Part model, mm, in its own coordinate system. Face numbers are marked on the shaded views. Give positions to 0.01 mm unless a question says otherwise; leave off trailing zeros. Order: outer loops, then holes, each group sorted by start corner. A loop starts at its lowest first (then second) coordinate and runs counter-clockwise, first axis right, second up. Notation, with made-up numbers: (9.25, 84) -> (35.25, 84) arc R23 cw to (35.25, 113) -> close; hole circle Ø7 at (27.5, 15.25). An arc over 180 degrees is marked (long way). Write item = value, one per line. Start each with the question number.
(1) Saw through at D-D, the plane y = 1.55. State how many separate pieces and enclosed holes the cut face has, then the cut area to 3 significant figures.
(2) Two-plate mould, pull along Y, no slides. Class the marked faces 1 and 2: pulls with the +Y half, pulls with the -Y half, needs draft (parallel to the pull), parting line crosses it, or undercut.
(3) Saw through at C-C, the plane x = 5. List the corners of the cut face in (y, z), then the cut area to 3 significant figures.
(4) Saw through at B-B, the plane z = 0. List the corners of the cut face in (x, y), then the cut area to 3 significant figures.
(5) Probe line 1 along Z through (x, y) = (160, 1); line 2 along Z through (x, y) = (172.5, 1.1); line 3 along X through (y, z) = (1.6, 4.5). List the from-to ranges inside material, lowest first. Write a range as from..to.
(6) Flat gauge pins, fed straight in: pin 1 (1 mm diameter, centred on y = 1.5, z = 10.5, fed in from -X); pin 2 (0.5 mm diameter, centred on y = 1.5, z = -3.5, fed in from +X); pin 3 (12.5 mm diameter, centred on x = 231.5, z = 2, fed in from +Y). Where does each tip first touch, or does it go through?
(7) Saw through at A-A, the plane x = 220. List the corners of the cut face in (y, z).
from build123d import *

# Parameters (mm, degrees)
BOSS_EXTRUDE1_DEPTH = 1.9
BOSS_EXTRUDE3_DEPTH = 0.95
SKETCH2_W           = 2
SKETCH2_H           = 5
BOSS_EXTRUDE2_DEPTH = 0.95


with BuildPart() as part:
    # Sketch1 → Boss-Extrude1 (new body)
    with BuildSketch(Plane(origin=(0, 0, 0), x_dir=(1, 0, 0), z_dir=(0, 1, 0))):
        with BuildLine():
            Line((0, -7.5), (0, -12.5))
            Line((0, -12.5), (210, -12.5))
            Line((210, -12.5), (210, 12.5))
            Line((210, 12.5), (0, 12.5))
            Line((0, 12.5), (0, 7.5))
            ThreePointArc((0, 7.5), (1.26826484, 7.391989197), (2.5, 7.071067812))
            ThreePointArc((2.5, 7.071067812), (12.5, 0), (2.5, -7.071067812))
            ThreePointArc((2.5, -7.071067812), (1.26826484, -7.391989197), (0, -7.5))
        make_face()
        with BuildLine():
            ThreePointArc((37.5, 7.071067812), (40, 7.5), (42.5, 7.071067812))
            ThreePointArc((42.5, 7.071067812), (45, 7.5), (47.5, 7.071067812))
            ThreePointArc((47.5, 7.071067812), (50, 7.5), (52.5, 7.071067812))
            ThreePointArc((52.5, 7.071067812), (55, 7.5), (57.5, 7.071067812))
            ThreePointArc((57.5, 7.071067812), (60, 7.5), (62.5, 7.071067812))
            ThreePointArc((62.5, 7.071067812), (65, 7.5), (67.5, 7.071067812))
            ThreePointArc((67.5, 7.071067812), (70, 7.5), (72.5, 7.071067812))
            ThreePointArc((72.5, 7.071067812), (75, 7.5), (77.5, 7.071067812))
            ThreePointArc((77.5, 7.071067812), (87.5, 0), (77.5, -7.071067812))
            ThreePointArc((77.5, -7.071067812), (75, -7.5), (72.5, -7.071067812))
            ThreePointArc((72.5, -7.071067812), (70, -7.5), (67.5, -7.071067812))
            ThreePointArc((67.5, -7.071067812), (65, -7.5), (62.5, -7.071067812))
            ThreePointArc((62.5, -7.071067812), (60, -7.5), (57.5, -7.071067812))
            ThreePointArc((57.5, -7.071067812), (55, -7.5), (52.5, -7.071067812))
            ThreePointArc((52.5, -7.071067812), (50, -7.5), (47.5, -7.071067812))
            ThreePointArc((47.5, -7.071067812), (45, -7.5), (42.5, -7.071067812))
            ThreePointArc((42.5, -7.071067812), (40, -7.5), (37.5, -7.071067812))
            ThreePointArc((37.5, -7.071067812), (27.5, 0), (37.5, 7.071067812))
        make_face(mode=Mode.SUBTRACT)
        with BuildLine():
            ThreePointArc((102.5, 7.071067812), (105, 7.5), (107.5, 7.071067812))
            ThreePointArc((107.5, 7.071067812), (110, 7.5), (112.5, 7.071067812))
            ThreePointArc((112.5, 7.071067812), (115, 7.5), (117.5, 7.071067812))
            ThreePointArc((117.5, 7.071067812), (120, 7.5), (122.5, 7.071067812))
            ThreePointArc((122.5, 7.071067812), (125, 7.5), (127.5, 7.071067812))
            ThreePointArc((127.5, 7.071067812), (130, 7.5), (132.5, 7.071067812))
            ThreePointArc((132.5, 7.071067812), (135, 7.5), (137.5, 7.071067812))
            ThreePointArc((137.5, 7.071067812), (147.5, 0), (137.5, -7.071067812))
            ThreePointArc((137.5, -7.071067812), (135, -7.5), (132.5, -7.071067812))
            ThreePointArc((132.5, -7.071067812), (130, -7.5), (127.5, -7.071067812))
            ThreePointArc((127.5, -7.071067812), (125, -7.5), (122.5, -7.071067812))
            ThreePointArc((122.5, -7.071067812), (120, -7.5), (117.5, -7.071067812))
            ThreePointArc((117.5, -7.071067812), (115, -7.5), (112.5, -7.071067812))
            ThreePointArc((112.5, -7.071067812), (110, -7.5), (107.5, -7.071067812))
            ThreePointArc((107.5, -7.071067812), (105, -7.5), (102.5, -7.071067812))
            ThreePointArc((102.5, -7.071067812), (92.5, 0), (102.5, 7.071067812))
        make_face(mode=Mode.SUBTRACT)
        with BuildLine():
            ThreePointArc((162.5, 7.071067812), (165, 7.5), (167.5, 7.071067812))
            ThreePointArc((167.5, 7.071067812), (170, 7.5), (172.5, 7.071067812))
            ThreePointArc((172.5, 7.071067812), (175, 7.5), (177.5, 7.071067812))
            ThreePointArc((177.5, 7.071067812), (180, 7.5), (182.5, 7.071067812))
            ThreePointArc((182.5, 7.071067812), (185, 7.5), (187.5, 7.071067812))
            ThreePointArc((187.5, 7.071067812), (190, 7.5), (192.5, 7.071067812))
            ThreePointArc((192.5, 7.071067812), (195, 7.5), (197.5, 7.071067812))
            ThreePointArc((197.5, 7.071067812), (207.5, 0), (197.5, -7.071067812))
            ThreePointArc((197.5, -7.071067812), (195, -7.5), (192.5, -7.071067812))
            ThreePointArc((192.5, -7.071067812), (190, -7.5), (187.5, -7.071067812))
            ThreePointArc((187.5, -7.071067812), (185, -7.5), (182.5, -7.071067812))
            ThreePointArc((182.5, -7.071067812), (180, -7.5), (177.5, -7.071067812))
            ThreePointArc((177.5, -7.071067812), (175, -7.5), (172.5, -7.071067812))
            ThreePointArc((172.5, -7.071067812), (170, -7.5), (167.5, -7.071067812))
            ThreePointArc((167.5, -7.071067812), (165, -7.5), (162.5, -7.071067812))
            ThreePointArc((162.5, -7.071067812), (152.5, 0), (162.5, 7.071067812))
        make_face(mode=Mode.SUBTRACT)
    extrude(amount=BOSS_EXTRUDE1_DEPTH)

    # Sketch1<3> → Boss-Extrude3 (add)
    with BuildSketch(Plane(origin=(0, 0, 0), x_dir=(1, 0, 0), z_dir=(0, 1, 0))):
        with BuildLine():
            Line((210, -12.5), (245, -12.5))
            ThreePointArc((245, -12.5), (257.5, 0), (245, 12.5))
            Line((245, 12.5), (210, 12.5))
            Line((210, 12.5), (210, -12.5))
        make_face()
        with BuildLine():
            ThreePointArc((222.5, -7.071067812), (212.5, 0), (222.5, 7.071067812))
            ThreePointArc((222.5, 7.071067812), (225, 7.5), (227.5, 7.071067812))
            ThreePointArc((227.5, 7.071067812), (230, 7.5), (232.5, 7.071067812))
            ThreePointArc((232.5, 7.071067812), (235, 7.5), (237.5, 7.071067812))
            ThreePointArc((237.5, 7.071067812), (240, 7.5), (242.5, 7.071067812))
            ThreePointArc((242.5, 7.071067812), (252.5, 0), (242.5, -7.071067812))
            ThreePointArc((242.5, -7.071067812), (240, -7.5), (237.5, -7.071067812))
            ThreePointArc((237.5, -7.071067812), (235, -7.5), (232.5, -7.071067812))
            ThreePointArc((232.5, -7.071067812), (230, -7.5), (227.5, -7.071067812))
            ThreePointArc((227.5, -7.071067812), (225, -7.5), (222.5, -7.071067812))
        make_face(mode=Mode.SUBTRACT)
    extrude(amount=BOSS_EXTRUDE3_DEPTH)

    # Sketch2 → Boss-Extrude2 (add)
    with BuildSketch(Plane(origin=(0, 0, 0), x_dir=(1, 0, 0), z_dir=(0, 1, 0))):
        with Locations((-1, 10)):
            Rectangle(SKETCH2_W, SKETCH2_H)
        with Locations((-1, -10)):
            Rectangle(SKETCH2_W, SKETCH2_H)
    extrude(amount=BOSS_EXTRUDE2_DEPTH)


solid = part.part
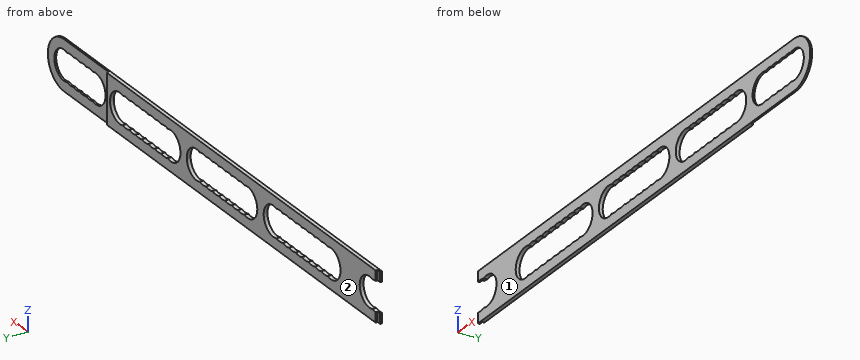
Results list:
q1.separate_pieces = 1
q1.enclosed_holes = 3
q1.area = 2,720 mm^2
q2.face_1 = pulls with the -Y half
q2.face_2 = pulls with the +Y half
q3.outline = (0, -12.5) -> (1.9, -12.5) -> (1.9, -7.5) -> (0, -7.5) -> close; (0, 7.5) -> (1.9, 7.5) -> (1.9, 12.5) -> (0, 12.5) -> close
q3.area = 19.0 mm^2
q4.outline = (12.5, 0) -> (27.5, 0) -> (27.5, 1.9) -> (12.5, 1.9) -> close; (87.5, 0) -> (92.5, 0) -> (92.5, 1.9) -> (87.5, 1.9) -> close; (147.5, 0) -> (152.5, 0) -> (152.5, 1.9) -> (147.5, 1.9) -> close; (207.5, 0) -> (212.5, 0) -> (212.5, 0.95) -> (210, 0.95) -> (210, 1.9) -> (207.5, 1.9) -> close; (252.5, 0) -> (257.5, 0) -> (257.5, 0.95) -> (252.5, 0.95) -> close
q4.area = 59.4 mm^2
q5.line_1 = -12.5..-7.5, 7.5..12.5
q5.line_2 = -12.5..-7.07, 7.07..12.5
q5.line_3 = 11..29, 86..94, 146..154, 206..210
q6.pin_1 = 0
q6.pin_2 = 210
q6.pin_3 = 0.95
q7.outline = (0, -12.5) -> (0.95, -12.5) -> (0.95, -7.5) -> (0, -7.5) -> close; (0, 7.5) -> (0.95, 7.5) -> (0.95, 12.5) -> (0, 12.5) -> close
